Design review of the part shown in the three views and the two pictorial views. Dimensions are in mm from the part's minimum x, y and z. Coordinates: 2 decimals unless noted, no trailing zeros. Order: outer loops, then holes, each group sorted by start corner. A loop starts at its lowest first (then second) coordinate and runs counter-clockwise, first axis right, second up. Notation, with made-up numbers: (29, 85.25) - (41, 85.25) arc R10 ccw to (41, 101.25) - close; hole circle Ø6 at (83, -0.5). An arc over 180 degrees is marked (long way). One line per item, written item: value. Start each with the question number.
(1) To check wall thickness, follow line 1 along X through (y, z) = (2.1, 24.13); line 2 along X through (y, z) = (0.45, 20.5); line 3 along Z through (x, y) = (76.2, 2.3) (3 decimals). State the ranges of each line that lie inside material, in increasing order.
(2) Consider section A-A on z = 24.13. Write out the cut boundary in (x, y) (1 decimal), then the cut area to 3 significant figures.
(3) Consider section C-C on y = 1.6. Count the separate pieces of the cut face and the enclosed holes in it, then the cut area to 3 significant figures.
(4) Consider section B-B on x = 25.4. Write out the cut boundary in (y, z) (3 decimals), then the cut area to 3 significant figures.
(5) Consider section D-D on z = 17.78. Write out the cut boundary in (x, y) (3 decimals).
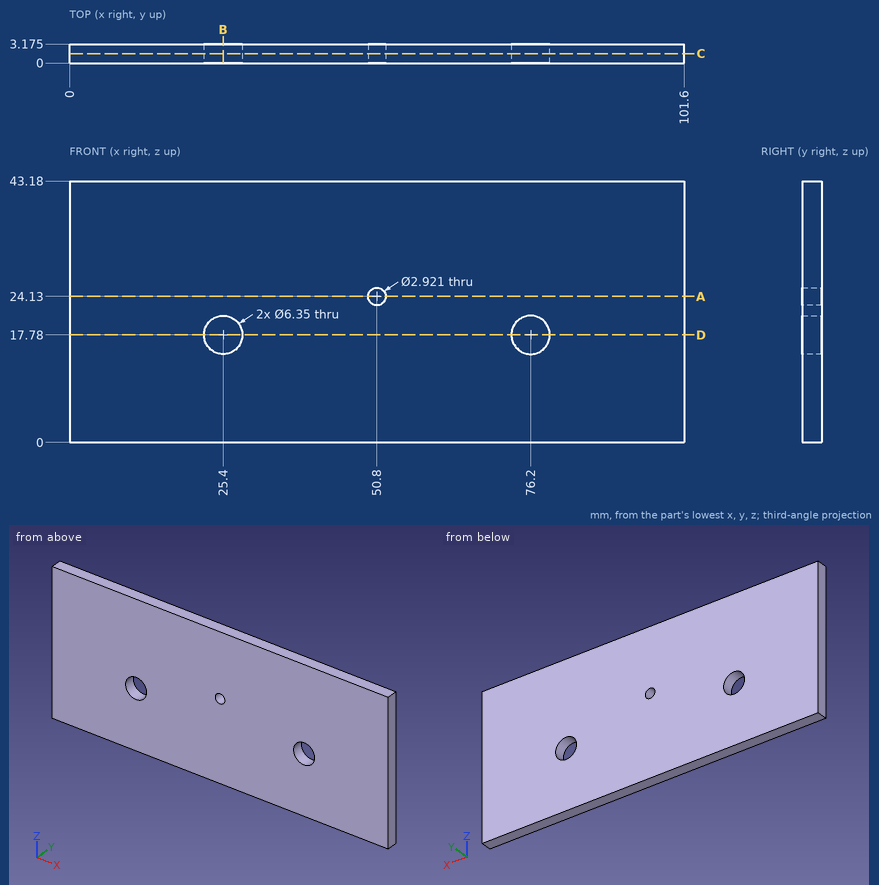
Geometry check:
1. line 1: x = 0 to 49.34, 52.26 to 101.6
1. line 2: x = 0 to 23.76, 27.04 to 74.56, 77.84 to 101.6
1. line 3: z = 0 to 14.605, 20.955 to 43.18
2. outline: (0, 0) - (49.3, 0) - (49.3, 3.2) - (0, 3.2) - close; (52.3, 0) - (101.6, 0) - (101.6, 3.2) - (52.3, 3.2) - close
2. area: 313 mm^2
3. separate pieces: 1
3. enclosed holes: 3
3. area: 4,320 mm^2
4. outline: (0, 0) - (3.175, 0) - (3.175, 14.605) - (0, 14.605) - close; (0, 20.955) - (3.175, 20.955) - (3.175, 43.18) - (0, 43.18) - close
4. area: 117 mm^2
5. outline: (0, 0) - (22.225, 0) - (22.225, 3.175) - (0, 3.175) - close; (28.575, 0) - (73.025, 0) - (73.025, 3.175) - (28.575, 3.175) - close; (79.375, 0) - (101.6, 0) - (101.6, 3.175) - (79.375, 3.175) - close
